Input: dimensioned drawing with shaded views. Units: mm. Origin: part minimum x, y, z. Coordinates: 2 decimals unless noted, no trailing zeros. Loops run counter-clockwise (first coordinate to the right, second up) from the corner with the lowest first, then second, coordinate; pieces in that order, holes last. Notation, with made-up numbers: M 41.25,-31.75 L 84.25,-31.75 A10 cw 84.25,-15.75 Z; hole C 79,-36 d2. An arc over 180 degrees is marked long. Write item = value, one per line. Start each with the question number.
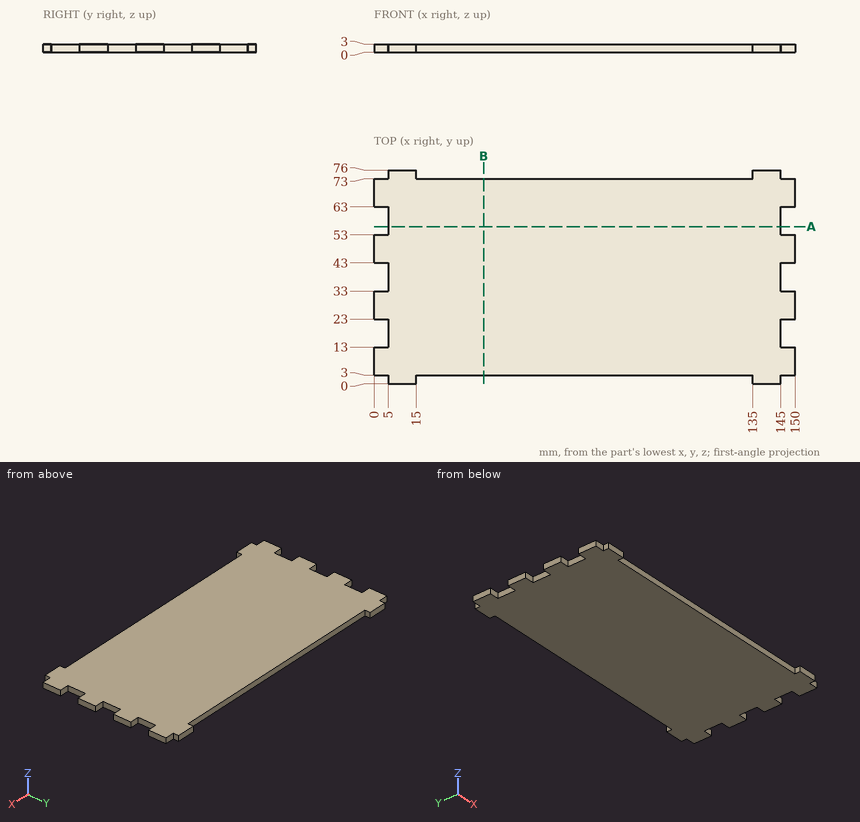
Item 1: Section query A-A (y = 56). Return the cut outline in (x, z).
Item 2: Section query B-B (x = 39). Return the cut outline in (y, z), plus the area to 3 significant figures.
Item 3: First-contact query: pin 1 (0.9 mm diameter, centred on x = 146.5, z = 2, fed in from +Y); pin 2 (10 mm diameter, centred on x = 55, y = 42, fed in from -Z); pin 3 (1.5 mm diameter, centred on x = 3, z = 2, fed in from -Y); pin 4 (1.5 mm diameter, centred on y = 17.5, z = 1, fed in from +X). Flat tips, straight axial feed; report the tip coordinate or a pass-through.
Item 4: Line query: line 1 (X direction, y = 20, z = 2); line 2 (Y direction, x = 130.5, z = 1.9). Output: solid intervals per line, ascending. Write a range as from..to.
Verdict:
q1.outline = M 5,0 L 145,0 L 145,3 L 5,3 Z
q2.outline = M 3,0 L 73,0 L 73,3 L 3,3 Z
q2.area = 210 mm2
q3.pin_1 = 73
q3.pin_2 = 0
q3.pin_3 = 3
q3.pin_4 = 145
q4.line_1 = 5..145
q4.line_2 = 3..73
